from build123d import *

# Parameters (mm, degrees)
BOX713_W        = 100
BOX713_H        = 100
BOX713_DEPTH    = 100
TUBE_R          = 16
TUBE_R_2        = 12
TUBE_DEPTH      = 40
CHAMFER002_SIZE = 2


with BuildPart() as krychle713:
    # Box713 → Box713 (new body)
    with BuildSketch(Plane(origin=(32, -54, -63), x_dir=(1, 0, 0), z_dir=(0, 0, 1))):
        with Locations((50, 50)):
            Rectangle(BOX713_W, BOX713_H)
    extrude(amount=BOX713_DEPTH)


with BuildPart() as cut530:
    # Tube → Tube (new body)
    with BuildSketch(Plane(origin=(75, 16, 42), x_dir=(1, 0, 0), z_dir=(0, -1, 0))):
        Circle(TUBE_R)
        Circle(TUBE_R_2, mode=Mode.SUBTRACT)
    extrude(amount=TUBE_DEPTH)

    # Chamfer002
    chamfer002_edges = [cut530.edges().sort_by_distance(p)[0] for p in [
        (59, -24, 42),
        (59, 16, 42),
    ]]
    chamfer(chamfer002_edges, length=CHAMFER002_SIZE)

    # Cut530: cut Krychle713
    add(krychle713.part, mode=Mode.SUBTRACT)


solid = cut530.part
Build history of the part. All positions in model axes, mm. Give positions to 0.01 mm unless a question says otherwise; leave off trailing zeros. Order: outer loops, then holes, each group sorted by start corner. A loop starts at its lowest first (then second) coordinate and runs counter-clockwise, first axis right, second up. Notation, with made-up numbers: M 5,5 L 21,5 A27 cw 21,34 Z; hole C 37,19.25 d3. An arc over 180 degrees is marked long. Use one line per item in the form item = value.
Q1. Slice it at A-A, the plane z = 42. Write the cut outline in (x, y), and give its area (3 significant figures).
Conclusion:
outline = M 59,-22 L 61,-24 L 63,-24 L 63,16 L 61,16 L 59,14 Z; M 87,-24 L 89,-24 L 91,-22 L 91,14 L 89,16 L 87,16 Z
area = 312 mm2
Q2. Pin check, flat tips, straight feed: P1, Ø8, axis at x = 86.5, y = -7.5, coming from the +Z side; P2, Ø6, axis at y = 1, z = 53, coming from the -X side; P3, Ø4, axis at x = 70, y = 1, coming from the -Z side. Stop position of each tip, or through.
Conclusion:
P1 = 56.13
P2 = 61.14
P3 = 51.75
Q3. Wall check: probe 1 along X at (y, z) = (-3.5, 42); probe 2 along Z at (x, y) = (75, -10.5); probe 3 along X at (y, z) = (-7.5, 50). Give the ranges that are in metal, low to high.
Conclusion:
probe_1 = 59 to 63, 87 to 91
probe_2 = 54 to 58
probe_3 = 61.14 to 66.06, 83.94 to 88.86
Q4. Slice it at C-C, the plane x = 75. Write the cut outline in (y, z).
Conclusion:
outline = M -24,54 L 16,54 L 16,56 L 14,58 L -22,58 L -24,56 Z
Q5. Slice it at B-B, the plane y = 1.5. Write the cut outline in (x, z).
Conclusion:
outline = M 59.8,37 L 64.09,37 A12 cw long 85.91,37 L 90.2,37 A16 ccw long Z
Q6. Pull direction X, two halves, no side cores. Call faces 1 (the cylindrical face through (75, -4, 54)), 2 (the flat face through (88, -4, 37)), 3 (the conical face through (75.388, 15.681, 56.314)): released by +X, released by -X, zero draft, split by the parting line, or undercut.
Conclusion:
face_1 = undercut
face_2 = zero draft
face_3 = split by the parting line
